from build123d import *

# Parameters (mm, degrees)
CROQUIS1_W              = 500
CROQUIS1_H              = 100
SALIENTE_EXTRUIR1_DEPTH = 40
VACIADO1_T              = -5
CROQUIS2_W              = 2.5
CROQUIS2_H              = 30
SALIENTE_EXTRUIR2_DEPTH = 100
CORTAR_EXTRUIR1_DEPTH   = 1.5
CORTAR_EXTRUIR2_DEPTH   = 5
CROQUIS5_R              = 10
CORTAR_EXTRUIR3_DEPTH   = 22.5
CROQUIS6_R              = 5
CORTAR_EXTRUIR4_DEPTH   = 281.5
CROQUIS7_W              = 70
CROQUIS7_H              = 65
CORTAR_EXTRUIR5_DEPTH   = 5
CHAFL_N1_SIZE           = 1
CHAFL_N2_SIZE           = 1


with BuildPart() as part:
    # Croquis1 → Saliente-Extruir1 (new body)
    with BuildSketch(Plane(origin=(0, 0, 0), x_dir=(1, 0, 0), z_dir=(0, 1, 0))):
        Rectangle(CROQUIS1_W, CROQUIS1_H)
    extrude(amount=SALIENTE_EXTRUIR1_DEPTH)

    # Vaciado1
    vaciado1_openings = [part.faces().sort_by_distance(p)[0] for p in [
        (0, 20, -50),
        (0, 20, 50),
    ]]
    offset(amount=VACIADO1_T, openings=vaciado1_openings, kind=Kind.INTERSECTION)

    # Croquis2 → Saliente-Extruir2 (add)
    with BuildSketch(Plane.XY.offset(50)):
        with Locations((-123.75, 20)):
            Rectangle(CROQUIS2_W, CROQUIS2_H)
        with Locations((-121.25, 20)):
            Rectangle(CROQUIS2_W, CROQUIS2_H)
        with Locations((-1.25, 20)):
            Rectangle(CROQUIS2_W, CROQUIS2_H)
        with Locations((1.25, 20)):
            Rectangle(CROQUIS2_W, CROQUIS2_H)
        with Locations((121.25, 20)):
            Rectangle(CROQUIS2_W, CROQUIS2_H)
        with Locations((123.75, 20)):
            Rectangle(CROQUIS2_W, CROQUIS2_H)
    extrude(amount=-SALIENTE_EXTRUIR2_DEPTH)

    # Croquis3 → Cortar-Extruir1 (cut)
    with BuildSketch(Plane(origin=(0, 40, 0), x_dir=(1, 0, 0), z_dir=(0, 1, 0))):
        with BuildLine():
            Line((-250, 20.5), (-150, 20.5))
            ThreePointArc((-150, 20.5), (-129.5, 0), (-150, -20.5))
            Line((-150, -20.5), (-250, -20.5))
            Line((-250, -20.5), (-250, 20.5))
        make_face()
        with BuildLine():
            Line((250, 20.5), (150, 20.5))
            ThreePointArc((150, 20.5), (129.5, 0), (150, -20.5))
            Line((150, -20.5), (250, -20.5))
            Line((250, -20.5), (250, 20.5))
        make_face()
    extrude(amount=-CORTAR_EXTRUIR1_DEPTH, mode=Mode.SUBTRACT)

    # Croquis4 → Cortar-Extruir2 (cut)
    with BuildSketch(Plane(origin=(0, 38.5, 0), x_dir=(1, 0, 0), z_dir=(0, 1, 0))):
        with BuildLine():
            Line((-150, -1.5), (-220, -1.5))
            ThreePointArc((-220, -1.5), (-221.5, 0), (-220, 1.5))
            Line((-220, 1.5), (-150, 1.5))
            ThreePointArc((-150, 1.5), (-148.5, 0), (-150, -1.5))
        make_face()
        with BuildLine():
            Line((150, 1.5), (220, 1.5))
            ThreePointArc((220, 1.5), (221.5, 0), (220, -1.5))
            Line((220, -1.5), (150, -1.5))
            ThreePointArc((150, -1.5), (148.5, 0), (150, 1.5))
        make_face()
    extrude(amount=-CORTAR_EXTRUIR2_DEPTH, mode=Mode.SUBTRACT)

    # Croquis5 → Cortar-Extruir3 (cut)
    with BuildSketch(Plane(origin=(0, 40, 0), x_dir=(1, 0, 0), z_dir=(0, 1, 0))):
        with Locations(Location((-150, 35, 0), (0, 0, 270))):
            Circle(CROQUIS5_R)
    cortar_extruir3 = extrude(amount=-CORTAR_EXTRUIR3_DEPTH, mode=Mode.SUBTRACT)

    # Simetría1: Cortar-Extruir3 across plane
    add(cortar_extruir3.mirror(Plane(origin=(0, 0, 0), x_dir=(0, 0, 1), z_dir=(1, 0, 0))), mode=Mode.SUBTRACT)

    # Croquis6 → Cortar-Extruir4 (cut)
    with BuildSketch(Plane.ZY.offset(125)):
        with Locations((-42, 27)):
            Circle(CROQUIS6_R)
        with Locations((-27, 27)):
            Circle(CROQUIS6_R)
        with Locations((-27, 12)):
            Circle(CROQUIS6_R)
        with Locations((-42, 12)):
            Circle(CROQUIS6_R)
    extrude(amount=-CORTAR_EXTRUIR4_DEPTH, mode=Mode.SUBTRACT)

    # Croquis7 → Cortar-Extruir5 (cut)
    with BuildSketch(Plane(origin=(0, 40, 0), x_dir=(1, 0, 0), z_dir=(0, 1, 0))):
        with Locations((-61.25, 0)):
            Rectangle(CROQUIS7_W, CROQUIS7_H)
        with Locations((61.25, 0)):
            Rectangle(CROQUIS7_W, CROQUIS7_H)
    extrude(amount=-CORTAR_EXTRUIR5_DEPTH, mode=Mode.SUBTRACT)

    # Chaflán1
    chafl_n1_edges = [part.edges().sort_by_distance(p)[0] for p in [
        (-96.25, 40, 0),
        (-61.25, 40, 32.5),
        (-26.25, 40, 0),
        (-61.25, 40, -32.5),
        (61.25, 40, 32.5),
        (96.25, 40, 0),
        (61.25, 40, -32.5),
        (26.25, 40, 0),
    ]]
    chamfer(chafl_n1_edges, length=CHAFL_N1_SIZE)

    # Chaflán2
    chafl_n2_edges = [part.edges().sort_by_distance(p)[0] for p in [
        (-150, 40, -45),
        (150, 40, -45),
    ]]
    chamfer(chafl_n2_edges, length=CHAFL_N2_SIZE)


solid = part.part
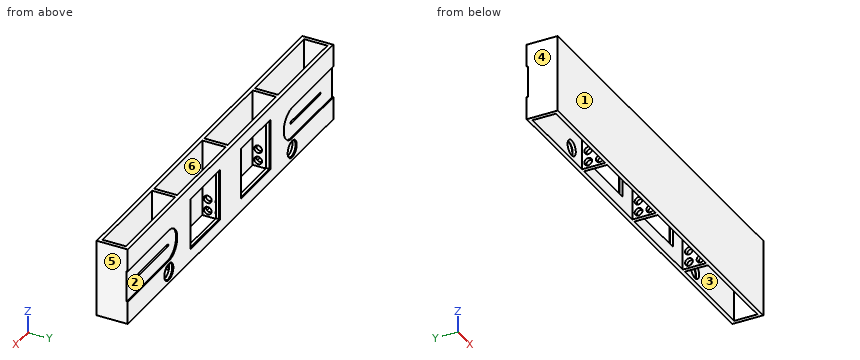
Work out the finished part from the listing and answer in its coordinate system (mm). Face numbers are marked on the shaded views. A direction names the side the tool comes from. Round coordinates to 2 decimals unless told otherwise and drop trailing zeros. Write each loop counter-clockwise with the first axis right and the second up, starting at its lowest first coordinate (ties: lowest second). Pieces come first, ordered by that corner, then holes. Notation, with made-up numbers: (-14, 44.5) - (8, 44.5) arc R12 ccw to (8, 50.5) - close; hole circle Ø7 at (5, 43.25). An arc over 180 degrees is marked (long way). Answer in a Markdown table with one row per item. Add a question column.
1. A cutting plane is placed at B-B, the plane z = 42. Determine the outline of the cut face in (x, y).
2. Given pin 1 (10 mm diameter, centred on x = -145, z = 8.5, fed in from +Y), flat-ended and moving along its own axis, determine where the tip first touches the part or whether it passes through.
3. A cutting plane is placed at A-A, the plane x = 44.5. Determine the outline of the cut face in (y, z), and give its area (3 significant figures).
4. Find the intervals of material crossed by line 1 along X through (y, z) = (36.7, -35); line 2 along X through (y, z) = (16, 33.5); line 3 along Y through (x, z) = (121, -42), in increasing order. Write a range as from..to.
5. The mould has two halves that part along X. Classify the marked faces 4, 5 and 6: +X half, -X half, draft (parallel to the pull), parting line (faces both ways), or undercut.
6. A cutting plane is placed at C-C, the plane x = -185.5. Determine the outline of the cut face in (y, z).
7. For the marked faces 1, 2 and 3, determine the directions among +Z, -Z, +X, -X, +Y, -Y from which every point of the face is accessible in a straight line to the end or side of a thin tool.
8. A cutting plane is placed at D-D, the plane z = 8. Count the separate pieces of the cut face and the enclosed holes in it, and give its area (3 significant figures).
Worked out:
| question | item | result |
|---|---|---|
| 1 | outline | (-250, 0) - (250, 0) - (250, 40) - (-250, 40) - close; hole (-245, 5) - (-125, 5) - (-125, 35) - (-245, 35) - close; hole (-120, 5) - (-2.5, 5) - (-2.5, 35) - (-120, 35) - close; hole (2.5, 5) - (120, 5) - (120, 35) - (2.5, 35) - close; hole (125, 5) - (245, 5) - (245, 35) - (125, 35) - close |
| 2 | pin 1 | y = 38.5 |
| 3 | outline | (0, -50) - (5, -50) - (5, 50) - (0, 50) - close; (35, -50) - (40, -50) - (40, -33.5) - (39, -32.5) - (35, -32.5) - close; (35, 32.5) - (39, 32.5) - (40, 33.5) - (40, 50) - (35, 50) - close |
| 3 | area | 674 mm^2 |
| 4 | line 1 | -250..-160, -140..140, 160..250 |
| 4 | line 2 | -250..-245, -125..-120, -2.5..2.5, 120..125, 245..250 |
| 4 | line 3 | 0..7, 17..22, 32..40 |
| 5 | face 4 | -X half |
| 5 | face 5 | +X half |
| 5 | face 6 | undercut |
| 6 | outline | (0, -50) - (5, -50) - (5, 50) - (0, 50) - close; (35, -50) - (40, -50) - (40, -20.5) - (38.5, -20.5) - (38.5, -1.5) - (35, -1.5) - close; (35, 1.5) - (38.5, 1.5) - (38.5, 20.5) - (40, 20.5) - (40, 50) - (35, 50) - close |
| 7 | face 1 | +Z, -Z, +X, -X, -Y |
| 7 | face 2 | +X, +Y |
| 7 | face 3 | +Z, -Z |
| 8 | separate pieces | 1 |
| 8 | enclosed holes | 2 |
| 8 | area | 4,690 mm^2 |
